from build123d import *

# Parameters (mm, degrees)
F0_R     = 2.413
F1_DEPTH = 2.54
F2_R     = 1.397
F3_DEPTH = 2.541
F4_R     = 25.4


with BuildPart() as f1:
    # F0 (on Top) → F1 (new body)
    with BuildSketch(Plane.XY):
        with BuildLine():
            Line((12.7, 37.3346617284), (12.7, 50.8))
            ThreePointArc((12.7, 50.8), (0, 63.5), (-12.7, 50.8))
            Line((-12.7, 50.8), (-12.7, 37.3346617284))
            Line((-12.7, 37.3346617284), (-9.144, 37.3346617284))
            ThreePointArc((-9.144, 37.3346617284), (-6.731, 39.7476617284), (-4.318, 37.3346617284))
            Line((-4.318, 37.3346617284), (4.318, 37.3346617284))
            ThreePointArc((4.318, 37.3346617284), (6.731, 39.7476617284), (9.144, 37.3346617284))
            Line((9.144, 37.3346617284), (12.7, 37.3346617284))
        make_face()
        with Locations((-6.731, 50.7966617284)):
            Circle(F0_R, mode=Mode.SUBTRACT)
        with Locations((6.731, 50.7966617284)):
            Circle(F0_R, mode=Mode.SUBTRACT)
        with BuildLine():
            ThreePointArc((2.3296350653, 0), (4.9703931971, 19.3740898835), (12.7, 37.3346617284))
            Line((12.7, 37.3346617284), (9.144, 37.3346617284))
            ThreePointArc((9.144, 37.3346617284), (6.731, 34.9216617284), (4.318, 37.3346617284))
            Line((4.318, 37.3346617284), (-4.318, 37.3346617284))
            ThreePointArc((-4.318, 37.3346617284), (-6.731, 34.9216617284), (-9.144, 37.3346617284))
            Line((-9.144, 37.3346617284), (-12.7, 37.3346617284))
            Line((-12.7, 37.3346617284), (-12.7, -37.3346617284))
            Line((-12.7, -37.3346617284), (-9.144, -37.3346617284))
            ThreePointArc((-9.144, -37.3346617284), (-6.731, -34.9216617284), (-4.318, -37.3346617284))
            Line((-4.318, -37.3346617284), (4.318, -37.3346617284))
            ThreePointArc((4.318, -37.3346617284), (6.731, -34.9216617284), (9.144, -37.3346617284))
            Line((9.144, -37.3346617284), (12.7, -37.3346617284))
            ThreePointArc((12.7, -37.3346617284), (4.9703931971, -19.3740898835), (2.3296350653, 0))
        make_face()
        with BuildLine():
            Line((-12.7, -37.3346617284), (-12.7, 37.3346617284))
            ThreePointArc((-12.7, 37.3346617284), (-23.0703649347, 0), (-12.7, -37.3346617284))
        make_face()
        with BuildLine():
            Line((12.7, -50.8), (12.7, -37.3346617284))
            Line((12.7, -37.3346617284), (9.144, -37.3346617284))
            ThreePointArc((9.144, -37.3346617284), (8.437248663, -39.0409103914), (6.731, -39.7476617284))
            Line((6.731, -39.7476617284), (6.731, -48.3836617284))
            ThreePointArc((6.731, -48.3836617284), (8.437248663, -49.0904130654), (9.144, -50.7966617284))
            ThreePointArc((9.144, -50.7966617284), (6.731, -53.2096617284), (4.318, -50.7966617284))
            Line((4.318, -50.7966617284), (-4.318, -50.7966617284))
            ThreePointArc((-4.318, -50.7966617284), (-8.437248663, -52.5029103914), (-6.731, -48.3836617284))
            Line((-6.731, -48.3836617284), (-6.731, -39.7476617284))
            ThreePointArc((-6.731, -39.7476617284), (-8.437248663, -39.0409103914), (-9.144, -37.3346617284))
            Line((-9.144, -37.3346617284), (-12.7, -37.3346617284))
            Line((-12.7, -37.3346617284), (-12.7, -50.8))
            ThreePointArc((-12.7, -50.8), (0, -63.5), (12.7, -50.8))
        make_face()
        with BuildLine():
            ThreePointArc((6.731, -39.7476617284), (5.024751337, -39.0409103914), (4.318, -37.3346617284))
            Line((4.318, -37.3346617284), (-4.318, -37.3346617284))
            ThreePointArc((-4.318, -37.3346617284), (-5.024751337, -39.0409103914), (-6.731, -39.7476617284))
            Line((-6.731, -39.7476617284), (-6.731, -48.3836617284))
            ThreePointArc((-6.731, -48.3836617284), (-5.024751337, -49.0904130654), (-4.318, -50.7966617284))
            Line((-4.318, -50.7966617284), (4.318, -50.7966617284))
            ThreePointArc((4.318, -50.7966617284), (5.024751337, -49.0904130654), (6.731, -48.3836617284))
            Line((6.731, -48.3836617284), (6.731, -39.7476617284))
        make_face()
    extrude(amount=F1_DEPTH)

    # F2 (on face) → F3 (cut, through all)
    with BuildSketch(Plane.XY.offset(2.54)):
        with BuildLine():
            ThreePointArc((0, -1.397), (0.9878281733, -0.9878281733), (1.397, 0))
            ThreePointArc((1.397, 0), (0.9878281733, 0.9878281733), (0, 1.397))
            Line((0, 1.397), (0, -1.397))
        make_face()
        with BuildLine():
            ThreePointArc((1.397, -12.7112130487), (0.9878281733, -11.7233848754), (0, -11.3142130487))
            ThreePointArc((0, -11.3142130487), (-0.9878281733, -13.699041222), (1.397, -12.7112130487))
        make_face()
        with BuildLine():
            ThreePointArc((1.397, 12.6887869513), (-0.9878281733, 13.6766151246), (0, 11.2917869513))
            ThreePointArc((0, 11.2917869513), (0.9878281733, 11.700958778), (1.397, 12.6887869513))
        make_face()
        with BuildLine():
            Line((0, -1.397), (0, 1.397))
            ThreePointArc((0, 1.397), (-1.397, 0), (0, -1.397))
        make_face()
        with BuildLine():
            ThreePointArc((0.9878281733, 45.0534899017), (0, 45.4626617284), (-0.9878281733, 45.0534899017))
            Line((-0.9878281733, 45.0534899017), (0, 44.0656617284))
            Line((0, 44.0656617284), (0.9878281733, 45.0534899017))
        make_face()
        with BuildLine():
            Line((0, 44.0656617284), (-0.9878281733, 45.0534899017))
            ThreePointArc((-0.9878281733, 45.0534899017), (-1.397, 44.0656617284), (-0.9878281733, 43.0778335551))
            Line((-0.9878281733, 43.0778335551), (0, 44.0656617284))
        make_face()
        with BuildLine():
            Line((0.9878281733, 45.0534899017), (0, 44.0656617284))
            Line((0, 44.0656617284), (0.9878281733, 43.0778335551))
            ThreePointArc((0.9878281733, 43.0778335551), (1.2906597069, 43.5310529734), (1.397, 44.0656617284))
            ThreePointArc((1.397, 44.0656617284), (1.2906597069, 44.6002704834), (0.9878281733, 45.0534899017))
        make_face()
        with BuildLine():
            Line((0.9878281733, 43.0778335551), (0, 44.0656617284))
            Line((0, 44.0656617284), (-0.9878281733, 43.0778335551))
            ThreePointArc((-0.9878281733, 43.0778335551), (0, 42.6686617284), (0.9878281733, 43.0778335551))
        make_face()
        with Locations((0, -44.0656617284)):
            Circle(F2_R)
    extrude(amount=-F3_DEPTH, mode=Mode.SUBTRACT)

    # F4
    f4_edges = [f1.edges().sort_by_distance(p)[0] for p in [
        (12.7, 37.334662, 1.27),
        (12.7, -37.334662, 1.27),
        (-12.7, 37.334662, 1.27),
        (-12.7, -37.334662, 1.27),
    ]]
    fillet(f4_edges, radius=F4_R)


solid = f1.part
Work out the finished part from the listing and answer in its coordinate system (mm). A direction names the side the tool comes from. Round coordinates to 2 decimals unless told otherwise and drop trailing zeros. Order: outer loops, then holes, each group sorted by start corner. A loop starts at its lowest first (then second) coordinate and runs counter-clockwise, first axis right, second up. Notation, with made-up numbers: M 50.5,67.25 L 103.5,67.25 A19 ccw 103.5,71.25 Z; hole C 52.25,25.5 d6. An arc over 180 degrees is marked long. Put each result on its own line as item: value. Start each with the question number.
Q1. Straight lines are drawn through the part: L1, parallel to X at y = 43.5, z = 1.05; L2, parallel to Y at x = -8, z = 0.3; L3, parallel to X at y = 48, z = 1.6. For each, find the intervals that lie inside material, in ascending order. Write a range as [from, to].
Q2. Section A-A, the plane x = -8 is taken. Write down the section's boundary in (y, z), and give its area (3 significant figures).
Q3. A flat-ended cylindrical pin translates along its axis: pin 1 (0.8 mm diameter, centred on y = -47, z = 1.5, fed in from -X). Find the tip coordinate at first contact, or state that the pin passes through.
Q4. Section B-B, the plane z = 1.9 is taken. Give the number of separate pieces and of enclosed holes in the cut face, and give its area (3 significant figures).
Q5. A tool of negligible diameter and unlimited length cuts with its end or side. For faces 1 (the flat face through (-12.7, 47, 1)), 2 (the flat face through (-12.7, -47, 1)), 3 (the cylindrical face through (12, -37.9, 1.3)), from which of +Z, -Z, +X, -X, +Y, -Y can it reach the whole face along a straight path? Write none if from no direction.
Q6. For a pull along X with two mould halves and no side action, classify faces 4 (the flat face through (-5, 1, 2.54)), 5 (the cylindrical face through (8.03, 52.83, 1.25)), 6 (the cylindrical face through (0.279, 63.497, 1.252)) as pulls with the +X half, pulls with the -X half, needs draft (parallel to the pull), parting line crosses it, or undercut.
Q7. Section C-C, the plane y = 20.5 is taken. Write down the section's boundary in (x, z).
Findings below:
1. L1: x = [-12.7, -1.28], [1.28, 12.7]
1. L2: y = [-60.66, -52.85], [-48.74, -39.39], [-35.28, 35.28], [39.39, 48.74], [52.85, 60.66]
1. L3: x = [-12.7, 12.7]
2. outline: M -60.66,0 L -52.85,0 L -52.85,2.54 L -60.66,2.54 Z; M -48.74,0 L -39.39,0 L -39.39,2.54 L -48.74,2.54 Z; M -35.28,0 L 35.28,0 L 35.28,2.54 L -35.28,2.54 Z; M 39.39,0 L 48.74,0 L 48.74,2.54 L 39.39,2.54 Z; M 52.85,0 L 60.66,0 L 60.66,2.54 L 52.85,2.54 Z
2. area: 266 mm^2
3. pin 1: stops at x = -12.7
4. separate pieces: 1
4. enclosed holes: 13
4. area: 2,910 mm^2
5. face 1: +Z, -Z, -X, +Y
5. face 2: +Z, -Z, -X, -Y
5. face 3: +Z, -Z, +X
6. face 4: needs draft
6. face 5: undercut
6. face 6: parting line crosses it
7. outline: M -20.11,0 L 5.29,0 L 5.29,2.54 L -20.11,2.54 Z
